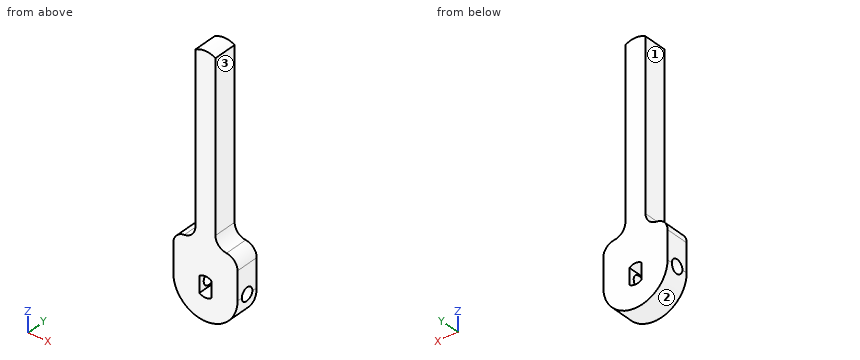
```python
from build123d import *

# Parameters (mm, degrees)
BOSS_EXTRU_1_DEPTH                        = 6
TROU_POUR_TARAUDAGE_POUR_TROU_TARAUD_M4_D = 3.3
CONG_1_R                                  = 3
CONG_2_R                                  = 3
CONG_3_R                                  = 3


with BuildPart() as part:
    # Esquisse1 → Boss.-Extru.1 (new body)
    with BuildSketch(Plane(origin=(0, 0, 0), x_dir=(1, 0, 0), z_dir=(0, 1, 0))):
        with BuildLine():
            Line((8, 0), (8, -10))
            Line((8, -10), (2.5, -10))
            Line((2.5, -10), (2.5, -54.330127019))
            ThreePointArc((2.5, -54.330127019), (0, -55), (-2.5, -54.330127019))
            Line((-2.5, -54.330127019), (-2.5, -10))
            Line((-2.5, -10), (-8, -10))
            Line((-8, -10), (-8, 0))
            ThreePointArc((-8, 0), (0, 8), (8, 0))
        make_face()
        with BuildLine():
            Line((1.5, 2), (1.5, -2))
            ThreePointArc((1.5, -2), (0, -2.5), (-1.5, -2))
            Line((-1.5, -2), (-1.5, 2))
            ThreePointArc((-1.5, 2), (0, 2.5), (1.5, 2))
        make_face(mode=Mode.SUBTRACT)
    extrude(amount=BOSS_EXTRU_1_DEPTH)

    # Trou pour taraudage pour trou taraudé M41 (through all)
    with Locations(Plane(origin=(8, 0, 0), x_dir=(0, 0, -1), z_dir=(1, 0, 0))):
        with Locations((0, 3)):
            Hole(TROU_POUR_TARAUDAGE_POUR_TROU_TARAUD_M4_D / 2)

    # Congé1
    cong_1_edges = [part.edges().sort_by_distance(p)[0] for p in [
        (-2.5, 3, 10),
    ]]
    fillet(cong_1_edges, radius=CONG_1_R)

    # Congé2
    cong_2_edges = [part.edges().sort_by_distance(p)[0] for p in [
        (-8, 3, 10),
        (2.5, 3, 10),
    ]]
    fillet(cong_2_edges, radius=CONG_2_R)

    # Congé3
    cong_3_edges = [part.edges().sort_by_distance(p)[0] for p in [
        (8, 3, 10),
    ]]
    fillet(cong_3_edges, radius=CONG_3_R)


solid = part.part
```
CAD build for the part. Positions are in the model's coordinates, mm. Face numbers are marked on the shaded views. A direction names the side the tool comes from. Round coordinates to 2 decimals unless told otherwise and drop trailing zeros. Loops run counter-clockwise (first coordinate to the right, second up) from the corner with the lowest first, then second, coordinate; pieces in that order, holes last. Notation, with made-up numbers: M -34.5,-23.75 L 21.5,-23.75 A12 ccw 21.5,-11.75 Z; hole C 32,-30.75 d6. An arc over 180 degrees is marked long. Return JSON: item names as keys, results as strings. Group by question number.
(1) Wall check: probe 1 along X at (y, z) = (5.25, 1.5); probe 2 along Y at (x, z) = (6.5, 0); probe 3 along X at (y, z) = (3, 43). Give the ranges that are in metal, low to high. Write a range as [from, to].
(2) Saw through at B-B, the plane z = 49.5. List the corners of the cut face in (x, y).
(3) Saw through at A-A, the plane x = 0. List the corners of the cut face in (y, z).
(4) Tool access for the marked faces 1, 2 and 3: list every direction of +Z, -Z, +X, -X, +Y, -Y with a clear straight run to the whole face (end or side of a thin tool).
(5) Drop flat-ended pins along their axis: P1, Ø1.8, axis at y = 4.5, z = 28, coming from the +X side; P2, Ø2, axis at y = 2, z = -1, coming from the +X side; P3, Ø1, axis at x = 6.5, y = 4.5, coming from the -Z side; P4, Ø1.2, axis at y = 2.5, z = -0.5, coming from the -X side. Give the stop position or say it passes through.
Answer list:
{
 "1": {"probe 1": "[-8, -1.5], [1.5, 8]", "probe 2": "[0, 1.35], [4.65, 6]", "probe 3": "[-2.5, 2.5]"},
 "2": {"outline": "M -2.5,0 L 2.5,0 L 2.5,6 L -2.5,6 Z"},
 "3": {"outline": "M 0,-8 L 6,-8 L 6,-2.5 L 0,-2.5 Z; M 0,2.5 L 6,2.5 L 6,55 L 0,55 Z"},
 "4": {"face 1": "+Z, -X, +Y, -Y", "face 2": "-Z, +Y, -Y", "face 3": "+Z, +X, +Y, -Y"},
 "5": {"P1": "x = 2.5", "P2": "x = 8", "P3": "z = -5.29", "P4": "through"}
}
